Input: part model. Units: mm. Frame: model coordinates. A direction names the side the tool comes from. Round coordinates to 2 decimals unless told otherwise and drop trailing zeros. Loops run counter-clockwise (first coordinate to the right, second up) from the corner with the lowest first, then second, coordinate; pieces in that order, holes last.
(1) Access query for faces 1 (the face through (1.17, -7.07, 1.88)), 2 (the face through (-13, 2.381, 2)). Directions: +Z, -Z, +X, -X, +Y, -Y. A direction counts if a zero-diameter tool reaches every point of the face in a straight line with its end or side. Return the directions, or none.
(2) Cut plane B-B, the plane x = 12. Output: boundary loops of the cut face in (y, z) (1 decimal), and give its area (3 significant figures).
(3) Line query: line 1 (X direction, y = 7, z = -111.5) (3 decimals); line 2 (Z direction, x = 7.5, y = 1.25) (3 decimals); line 3 (Y direction, x = -12, z = -47). Output: solid intervals per line, ascending.
(4) Cut plane A-A, the plane y = -5.5. Output: boundary loops of the cut face in (x, z).
(5) First-contact query: pin 1 Ø3 at (y, z) = (5.5, -34) entering from -X (3 decimals); pin 2 Ø4 at (y, z) = (2, 34) entering from +X; pin 3 Ø0.6 at (x, z) = (-15, 19) entering from -Y. Flat tips, straight axial feed; report the tip coordinate or a pass-through.
from build123d import *

# Parameters (mm, degrees)
F1_DEPTH = 146.05
F2_R     = 2.54
F3_R     = 2.54
F4_R     = 2.54
F6_DEPTH = 17.4635001
F8_DEPTH = 6.35


# Not quite as in the source:
# - ends of sketch curves that miss each other by under 0.0002 mm in the source are joined


with BuildPart() as f1:
    # F0 (on Top) → F1 (new body, symmetric)
    with BuildSketch(Plane.XY):
        with BuildLine():
            Line((15.875, 5.55625), (15.875, 8.73125))
            Line((15.875, 8.73125), (-15.875, 8.73125))
            Line((-15.875, 8.73125), (-15.875, -0.79375))
            Line((-15.875, -0.79375), (-12.7, -0.79375))
            ThreePointArc((-12.7, -0.79375), (-9.8710707302, -6.4481459867), (-3.9751, -8.73125))
            Line((-3.9751, -8.73125), (-3.96875, -8.73125))
            ThreePointArc((-3.96875, -8.73125), (1.9312218072, -6.4502821485), (4.7625, -0.79375))
            Line((4.7625, -0.79375), (7.9375, -0.79375))
            ThreePointArc((7.9375, -0.79375), (10.9883747468, 3.5285940665), (15.875, 5.55625))
        make_face()
    extrude(amount=F1_DEPTH, both=True)

    # F2
    f2_edges = [f1.edges().sort_by_distance(p)[0] for p in [
        (7.9375, -0.79375, 0),
    ]]
    fillet(f2_edges, radius=F2_R)

    # F3
    f3_edges = [f1.edges().sort_by_distance(p)[0] for p in [
        (-12.7, -0.79375, 0),
    ]]
    fillet(f3_edges, radius=F3_R)

    # F4
    f4_edges = [f1.edges().sort_by_distance(p)[0] for p in [
        (4.7625, -0.79375, 0),
    ]]
    fillet(f4_edges, radius=F4_R)

    # F5 (on face) → F6 (cut, through all)
    with BuildSketch(Plane(origin=(0, 8.73125, 0), x_dir=(-1, 0, 0), z_dir=(0, 1, 0))):
        Polygon((15.875, 146.05), (-15.875, 146.05), (15.875, 114.3), align=None)
        Polygon((15.875, -114.3), (-15.875, -146.05), (15.875, -146.05), align=None)
    extrude(amount=-F6_DEPTH, mode=Mode.SUBTRACT)

    # F7 (on face) → F8 (cut)
    with BuildSketch(Plane(origin=(0, 8.73125, 0), x_dir=(-1, 0, 0), z_dir=(0, 1, 0))):
        Polygon((9.525, 120.65), (9.525, -120.65), (15.875, -114.3), (15.875, 114.3), align=None)
    extrude(amount=-F8_DEPTH, mode=Mode.SUBTRACT)


solid = f1.part
Reported:
1. face 1: +Z, -Z, +X, -Y
1. face 2: +Z, -Z, -X, +Y
2. outline: (4.2, -142.2) - (8.7, -142.2) - (8.7, 142.2) - (4.2, 142.2) - close
2. area: 1,280 mm2
3. line 1: x = -9.525 to 15.875
3. line 2: z = -137.675 to 137.675
3. line 3: y = -3.49 to 2.38
4. outline: (-10.77, -119.41) - (2.83, -133.01) - (2.83, 133.01) - (-10.77, 119.41) - close
5. pin 1: stops at x = -9.525
5. pin 2: stops at x = 11.63
5. pin 3: stops at y = -0.79
